Input: part model. Units: mm. Frame: model coordinates. A direction names the side the tool comes from. Coordinates: 2 decimals unless noted, no trailing zeros. Write each loop counter-clockwise with the first axis right and the second up, starting at its lowest first coordinate (ties: lowest second). Pieces come first, ordered by that corner, then holes.
from build123d import *

# Parameters (mm, degrees)
F0_R     = 1.5
F0_R_2   = 2
F1_DEPTH = 3


with BuildPart() as f1:
    # F0 (on Top) → F1 (new body)
    with BuildSketch(Plane.XY):
        with BuildLine():
            Line((-60, -5), (-4.8989794856, -5))
            ThreePointArc((-4.8989794856, -5), (-7, 0), (-4.8989794856, 5))
            Line((-4.8989794856, 5), (-52, 5))
            Line((-52, 5), (-52, 3))
            Line((-52, 3), (-56, 3))
            Line((-56, 3), (-56, 5))
            Line((-56, 5), (-60, 5))
            Line((-60, 5), (-60, -5))
        make_face()
        with Locations((-30, 0)):
            Circle(F0_R, mode=Mode.SUBTRACT)
        with BuildLine():
            Line((-4.8989794856, -5), (4.8989794856, -5))
            ThreePointArc((4.8989794856, -5), (6.4534043883, -2.7117470016), (7, 0))
            ThreePointArc((7, 0), (6.4534043883, 2.7117470016), (4.8989794856, 5))
            Line((4.8989794856, 5), (-4.8989794856, 5))
            ThreePointArc((-4.8989794856, 5), (-7, 0), (-4.8989794856, -5))
        make_face()
        Circle(F0_R_2, mode=Mode.SUBTRACT)
        with BuildLine():
            ThreePointArc((4.8989794856, 5), (0, 7), (-4.8989794856, 5))
            Line((-4.8989794856, 5), (4.8989794856, 5))
        make_face()
        with BuildLine():
            ThreePointArc((-4.8989794856, -5), (0, -7), (4.8989794856, -5))
            Line((4.8989794856, -5), (-4.8989794856, -5))
        make_face()
        with BuildLine():
            Line((4.8989794856, -5), (60, -5))
            Line((60, -5), (60, 5))
            Line((60, 5), (59, 5))
            ThreePointArc((59, 5), (53, -1), (47, 5))
            Line((47, 5), (4.8989794856, 5))
            ThreePointArc((4.8989794856, 5), (6.4534043883, 2.7117470016), (7, 0))
            ThreePointArc((7, 0), (6.4534043883, -2.7117470016), (4.8989794856, -5))
        make_face()
    extrude(amount=F1_DEPTH)


solid = f1.part
Item 1: Section query D-D, the plane x = 0. Return loops of the section in (y, z).
Item 2: Pin query (flat end, axial travel): pin 1 Ø1.5 at (x, z) = (-23, 1.5) entering from +Y; pin 2 Ø3.5 at (x, y) = (-30, 0) entering from +Z. Return the tip coordinate at first contact, or that it passes through.
Item 3: Access query for faces 1 (the face through (-33, -5, 1)), 2 (the face through (-58, 5, 1)), 3 (the face through (26, 5, 1)). Directions: +Z, -Z, +X, -X, +Y, -Y. A direction counts if a zero-diameter tool reaches every point of the face in a straight line with its end or side. Return the directions, or none.
Item 4: Material intervals for line 1 (X direction, y = 4.75, z = 1.3); line 2 (X direction, y = 1, z = 2.3); line 3 (Y direction, x = -30, z = 2), sorted ascending.
Item 5: Section query B-B, the plane z = 1.8. Return loops of the section in (x, y).
Item 6: Section query C-C, the plane y = 0. Return loops of the section in (x, z).
Item 7: Section query A-A, the plane x = -30. Return loops of the section in (y, z), then the cut area to 3 significant figures.
The answers:
1. outline: (-7, 0) - (-2, 0) - (-2, 3) - (-7, 3) - close; (2, 0) - (7, 0) - (7, 3) - (2, 3) - close
2. pin 1: stops at y = 5
2. pin 2: stops at z = 3
3. face 1: +Z, -Z, -X, -Y
3. face 2: +Z, -Z, -X, +Y
3. face 3: +Z, -Z, +X, +Y
4. line 1: x = -60 to -56, -52 to 47.01, 58.99 to 60
4. line 2: x = -60 to -31.12, -28.88 to -1.73, 1.73 to 48.53, 57.47 to 60
4. line 3: y = -5 to -1.5, 1.5 to 5
5. outline: (-60, -5) - (-4.9, -5) arc R7 ccw to (4.9, -5) - (60, -5) - (60, 5) - (59, 5) arc R6 cw to (47, 5) - (4.9, 5) arc R7 ccw to (-4.9, 5) - (-52, 5) - (-52, 3) - (-56, 3) - (-56, 5) - (-60, 5) - close; hole circle Ø3 at (-30, 0); hole circle Ø4 at (0, 0)
6. outline: (-60, 0) - (-31.5, 0) - (-31.5, 3) - (-60, 3) - close; (-28.5, 0) - (-2, 0) - (-2, 3) - (-28.5, 3) - close; (2, 0) - (49.68, 0) - (49.68, 3) - (2, 3) - close; (56.32, 0) - (60, 0) - (60, 3) - (56.32, 3) - close
7. outline: (-5, 0) - (-1.5, 0) - (-1.5, 3) - (-5, 3) - close; (1.5, 0) - (5, 0) - (5, 3) - (1.5, 3) - close
7. area: 21.0 mm2
